Work out the finished part from the listing and answer in its coordinate system (mm). A direction names the side the tool comes from. Round coordinates to 2 decimals unless told otherwise and drop trailing zeros. Order: outer loops, then holes, each group sorted by start corner. A loop starts at its lowest first (then second) coordinate and runs counter-clockwise, first axis right, second up. Notation, with made-up numbers: (-20.5, 85) -> (3.5, 85) arc R14 ccw to (3.5, 97) -> close; hole circle Ø5 at (56, -27.5). An arc over 180 degrees is marked (long way). Use one line per item in the form item = value.
```python
from build123d import *

# Parameters (mm, degrees)
F0_R        = 7.5
F1_DEPTH    = 75
F2_T        = -1
F4_DEPTH    = 25
F6_D        = 1.5
F6_DEPTH    = 25
F6_TIP      = 0.4506454643
F5_R        = 0.8075633059
F5_R_2      = 0.5172212245
F5_R_3      = 0.4893329223
F7_DEPTH    = 25
F9_START    = -15
F8_R        = 9.5
F8_R_2      = 7.5
F9_DEPTH    = 37
F10_START   = -1.5
F9_FACE_R   = 9.5
F9_FACE_R_2 = 7.5
F10_DEPTH   = 34.1
F12_DEPTH   = 37
F13_W       = 3.3348486101
F13_H       = 34.1
F13_W_2     = 5
F14_DEPTH   = 25
F16_D       = 1.5
F16_DEPTH   = 200
F16_TIP     = 0.4506454643
F17_R       = 0.6
F18_DEPTH   = 2
F19_SIZE    = 0.2
F20_R       = 0.6
F21_DEPTH   = 3.5
F22_SIZE    = 0.2


with BuildPart() as f1:
    # F0 (on Top) → F1 (new body)
    with BuildSketch(Plane.XY):
        Circle(F0_R)
    extrude(amount=F1_DEPTH)

    # F2
    f2_openings = [f1.faces().sort_by_distance(p)[0] for p in [
        (0, 0, 75),
    ]]
    offset(amount=F2_T, openings=f2_openings)

    # F3 (on face) → F4 (cut)
    with BuildSketch(Plane(origin=(0, 0, 0), x_dir=(1, 0, 0), z_dir=(0, 0, -1))):
        with BuildLine():
            Line((-5.0392321942, 2), (5.0392321942, 2))
            ThreePointArc((5.0392321942, 2), (0, 5.421610564), (-5.0392321942, 2))
        make_face()
        with BuildLine():
            ThreePointArc((-5.0392321942, -2), (0, -5.421610564), (5.0392321942, -2))
            Line((5.0392321942, -2), (-5.0392321942, -2))
        make_face()
    extrude(amount=-F4_DEPTH, mode=Mode.SUBTRACT)

    # F6
    with Locations(Plane(origin=(0, 0, 0), x_dir=(1, 0, 0), z_dir=(0, 0, -1))):
        with Locations((0, 0)):
            Hole(F6_D / 2, depth=F6_DEPTH)
            with Locations((0, 0, -(F6_DEPTH + F6_TIP / 2))):  # 118° drill point
                Cone(0, F6_D / 2, F6_TIP, mode=Mode.SUBTRACT)

    # F5 (on face) → F7 (cut)
    with BuildSketch(Plane(origin=(0, 0, 0), x_dir=(1, 0, 0), z_dir=(0, 0, -1))):
        Circle(F5_R)
        with Locations((-3.9731087163, 0)):
            Circle(F5_R_2)
        with Locations((4.63699596, 0)):
            Circle(F5_R_3)
    extrude(amount=-F7_DEPTH, mode=Mode.SUBTRACT)

    # F8 (on face) → F9 (join)
    with BuildSketch(Plane.XY.offset(75).offset(F9_START)):
        Circle(F8_R)
        Circle(F8_R_2, mode=Mode.SUBTRACT)
    extrude(amount=-F9_DEPTH)

    # F9_face (on face) → F10 (cut)
    with BuildSketch(Plane.XY.offset(60).offset(F10_START)):
        Circle(F9_FACE_R)
        Circle(F9_FACE_R_2, mode=Mode.SUBTRACT)
    extrude(amount=-F10_DEPTH, mode=Mode.SUBTRACT)

    # F11 (on face) → F12 (join)
    with BuildSketch(Plane.XY.offset(60)):
        with BuildLine():
            ThreePointArc((2.5, -9.1651513899), (0, -9.5), (-2.5, -9.1651513899))
            Line((-2.5, -9.1651513899), (-2.5, -12.5))
            Line((-2.5, -12.5), (2.5, -12.5))
            Line((2.5, -12.5), (2.5, -9.1651513899))
        make_face()
        with BuildLine():
            Line((-2.5, 12.5), (-2.5, 9.1651513899))
            ThreePointArc((-2.5, 9.1651513899), (0, 9.5), (2.5, 9.1651513899))
            Line((2.5, 9.1651513899), (2.5, 12.5))
            Line((2.5, 12.5), (-2.5, 12.5))
        make_face()
    extrude(amount=-F12_DEPTH)

    # F13 (on face) → F14 (cut)
    with BuildSketch(Plane.YZ.offset(2.5)):
        with Locations((10.832575695, 41.45)):
            Rectangle(F13_W, F13_H)
        with Locations((-11.1832837015, 41.45)):
            Rectangle(F13_W_2, F13_H)
    extrude(amount=-F14_DEPTH, mode=Mode.SUBTRACT)

    # F16
    with Locations(Plane.XY.offset(60)):
        with Locations((0, 10.4414262056)):
            Hole(F16_D / 2, depth=F16_DEPTH)
            with Locations((0, 0, -(F16_DEPTH + F16_TIP / 2))):  # 118° drill point
                Cone(0, F16_D / 2, F16_TIP, mode=Mode.SUBTRACT)

    # F17 (on face) → F18 (join)
    with BuildSketch(Plane.XY.offset(60)):
        with Locations((0, -10.3)):
            Circle(F17_R)
    extrude(amount=F18_DEPTH)

    # F19
    f19_edges = [f1.edges().sort_by_distance(p)[0] for p in [
        (-0.6, -10.3, 62),
    ]]
    chamfer(f19_edges, length=F19_SIZE)

    # F20 (on face) → F21 (join)
    with BuildSketch(Plane.XY.offset(24.4)):
        with Locations((0.2855480707, -10.4)):
            Circle(F20_R)
    extrude(amount=-F21_DEPTH)

    # F22
    f22_edges = [f1.edges().sort_by_distance(p)[0] for p in [
        (-0.314452, -10.4, 20.9),
    ]]
    chamfer(f22_edges, length=F22_SIZE)


solid = f1.part
```
Item 1: Flat-ended cylindrical pins translate along their axes: P1, Ø10.5, axis at x = -2, y = -1.5, coming from the +Z side; P2, Ø0.6, axis at x = 0.5, y = -10.5, coming from the -Z side; P3, Ø0.8, axis at y = -10.5, z = 59.5, coming from the +X side; P4, Ø1, axis at x = -0.5, y = 5, coming from the +Z side. Find the tip coordinate at first contact, or state that the pin passes through.
Findings:
P1 = 75
P2 = 20.9
P3 = 2.5
P4 = 1
Item 2: The part is cut by section B-B, the plane z = 30. Give the vertices of the cut face in (x, y), and give its area (3 significant figures).
Findings:
outline = circle Ø15 at (0, 0); hole circle Ø13 at (0, 0)
area = 44.0 mm^2
Item 3: Consider line 1 along Y through (x, z) = (0, 59.35); line 2 along Z through (x, y) = (4, 8.5); line 3 along X through (y, z) = (-0.25, 54.5). Determine where each line is inside the solid, lowest interval first.
Findings:
line_1 = -12.5 to -6.5, 6.5 to 9.69, 11.19 to 12.5
line_2 = 23 to 24.4, 58.5 to 60
line_3 = -7.5 to -6.5, 6.5 to 7.5
Item 4: For faces 1 (the cylindrical face through (-5.158, -3.955, 37.482)), 2 (the flat face through (0, -12.5, 59)), 3 (the flat face through (-4.3, -6.4, 58.5)), 4 (the cylindrical face through (-7.493, 0.33, 11.339)), 5 (the flat face through (-2.5, -11, 59)), determine the directions among +Z, -Z, +X, -X, +Y, -Y from which every point of the face is accessible in a straight line to the end or side of a thin tool.
Findings:
face_1 = +Z
face_2 = +Z, -Z, +X, -X, -Y
face_3 = none
face_4 = -Z
face_5 = +Z, -Z, -X, -Y
Item 5: The part is cut by section A-A, the plane y = -3.5. Give the vertices of the cut face in (x, z).
Findings:
outline = (-8.83, 23) -> (-6.63, 23) -> (-6.63, 0) -> (-4.14, 0) -> (-4.14, 1) -> (-5.48, 1) -> (-5.48, 75) -> (-6.63, 75) -> (-6.63, 60) -> (-8.83, 60) -> (-8.83, 58.5) -> (-6.63, 58.5) -> (-6.63, 24.4) -> (-8.83, 24.4) -> close; (4.14, 0) -> (6.63, 0) -> (6.63, 23) -> (8.83, 23) -> (8.83, 24.4) -> (6.63, 24.4) -> (6.63, 58.5) -> (8.83, 58.5) -> (8.83, 60) -> (6.63, 60) -> (6.63, 75) -> (5.48, 75) -> (5.48, 1) -> (4.14, 1) -> close
Item 6: Determine the mould class of faces 6 (the cylindrical face through (9.5, -0.17, 23.71)), 7 (the cylindrical face through (0.55, 10.95, 23.69)), 8 (the flat face through (-2.5, 11, 24)) for opening direction X: released by +X, released by -X, zero draft, split by the parting line, or undercut.
Findings:
face_6 = released by +X
face_7 = undercut
face_8 = released by -X
